Here's how the part is built. I have some questions about the finished solid (model axes, mm). A direction names the side the tool comes from. Round coordinates to 2 decimals unless told otherwise and drop trailing zeros. Order: outer loops, then holes, each group sorted by start corner. A loop starts at its lowest first (then second) coordinate and runs counter-clockwise, first axis right, second up. Notation, with made-up numbers: (-3, 5.25) -> (34, 5.25) arc R14 cw to (34, 22.25) -> close; hole circle Ø11 at (18.5, -7.5). An arc over 180 degrees is marked (long way). One line per item, written item: value.
Autodesk Inventor part; units mm, degrees
ref_plane "YZ Plane" through (0, 0, 0) normal (1, 0, 0) x (0, 1, 0)
ref_plane "XZ Plane" through (0, 0, 0) normal (0, 1, 0) x (-1, 0, 0)
ref_plane "XY Plane" through (0, 0, 0) normal (0, 0, 1) x (1, 0, 0)
sketch "Sketch1" plane through (0, 0, 0) normal (0, 0, 1) x (1, 0, 0)
  line L0 (-12.7, -12.7) -> (12.7, -12.7)
  line L1 (12.7, -12.7) -> (12.7, 12.7)
  line L2 (12.7, 12.7) -> (-12.7, 12.7)
  line L3 (-12.7, 12.7) -> (-12.7, -12.7)
  line L4 (-12.7, -12.7) -> (12.7, 12.7) construction
  line L5 (12.7, -12.7) -> (-12.7, 12.7) construction
  line L6 (-11.1125, 11.1125) -> (11.1125, 11.1125)
  line L7 (11.1125, 11.1125) -> (11.1125, -11.1125)
  line L8 (11.1125, -11.1125) -> (-11.1125, -11.1125)
  line L9 (-11.1125, -11.1125) -> (-11.1125, 11.1125)
  point P0 (0, 0)
  dimension "width" = 25.4
  dimension "height" = 25.4
  dimension "thickness" = 1.5875
extrude "Extrusion1" add sketch "Sketch1" along normal mid plane 431.8
sketch "Sketch3" plane through (-12.7, 12.7, 215.9) normal (0, 1, 0) x (1, 0, 0)
  line L0 (0, 431.8) -> (0, 0) construction
  line L1 (25.4, 0) -> (0, 0) construction
  line L2 (25.4, 431.8) -> (25.4, 0) construction
  line L3 (0, 431.8) -> (25.4, 431.8) construction
  line L4 (0, 0) -> (0, 431.8) construction
  line L5 (0, 0) -> (25.4, 17.7853)
  line L6 (25.4, 431.8) -> (25.4, 0) construction
  line L7 (0, 0) -> (25.4, 0) construction
  line L8 (0, 0) -> (25.4, 0)
  line L9 (25.4, 0) -> (25.4, 17.7853)
  line L10 (0, 431.8) -> (25.4, 395.525)
  line L11 (25.4, 431.8) -> (0, 431.8) construction
  line L12 (0, 431.8) -> (25.4, 431.8)
  line L13 (25.4, 431.8) -> (25.4, 395.525)
  point P0 (12.7, 215.9)
  dimension "d12" = 55
extrude "Extrusion3" cut sketch "Sketch3" against normal through all
sketch "Sketch4" plane through (-12.7, 12.7, 215.9) normal (0, 1, 0) x (1, 0, 0)
  line L0 (25.4, 17.7853) -> (0, 0) construction
  line L1 (0, 0) -> (0, 431.8) construction
  line L2 (0, 431.8) -> (25.4, 395.525) construction
  line L3 (25.4, 395.525) -> (25.4, 17.7853) construction
  point P0 (12.7, 215.9)
  point P1 (12.7, 19.05)
  point P2 (12.7, 31.75)
  point P3 (12.7, 44.45)
  point P4 (12.7, 57.15)
  point P5 (12.7, 400.05)
  point P6 (12.7, 387.35)
  point P7 (12.7, 374.65)
  dimension "d13" = 19.05
  dimension "d16" = 12.7
  dimension "d28" = 31.75
  dimension "d31" = 12.7
hole "Hole1" at (0, 12.7, 196.85) at (0, 12.7, 184.15) at (0, 12.7, -158.75) at (0, 12.7, -171.45) at (0, 12.7, -184.15) direction (0, -1, 0) diameter 5.1054 end through all
sketch "Sketch5" plane through (-12.7, -12.7, 215.9) normal (-1, 0, 0) x (0, 0, 1)
  line L0 (-431.8, 0) -> (-431.8, 25.4) construction
  point P0 (-215.9, 12.7)
  point P1 (-241.3, 12.7)
  point P2 (-203.2, 12.7)
  point P3 (-431.8, 12.7)
  dimension "d36" = 38.1
  dimension "d37" = 190.5
hole "Hole2" at (-12.7, 0, -25.4) at (-12.7, 0, 12.7) direction (1, 0, 0) diameter 5.1054 end through all
sketch "Sketch6" plane through (-12.7, 12.7, 215.9) normal (0, 1, 0) x (1, 0, 0)
  line L0 (25.4, 395.525) -> (25.4, 17.7853) construction
  circle A0 centre (12.7, 374.65) radius 2.5527 construction
  point P0 (12.7, 215.9)
  point P1 (12.7, 222.25)
  point P2 (12.7, 190.5)
  dimension "d45" = 31.75
  dimension "d46" = 12.7
  dimension "d47" = 152.4
hole "Hole3" at (0, 12.7, -6.35) at (0, 12.7, 25.4) direction (0, -1, 0) diameter 5.1054 end through all
properties part number "CL-002" material "Aluminum 6061"
Q1. If we mould it in two halves opening along X, with no side actions, what happens to faces 1 (the face through (0, 12.7, -3)), 2 (the face through (11.112, 0, 6)), 3 (the face through (12.7, 0, 7))? For each: pulls with the +X half, pulls with the -X half, needs draft (parallel to the pull), parting line crosses it, or undercut.
Answers:
face 1: needs draft
face 2: undercut
face 3: pulls with the +X half
Q2. I need wall thicknesses on line 1 along Y through (x, z) = (-6, 48.5); line 2 along Y through (x, z) = (11.5, -25.4). Which ranges of each line are inside material? Lowest first, please.
Answers:
line 1: -12.7 to -11.11, 11.11 to 12.7
line 2: -12.7 to -2.55, 2.55 to 12.7
Q3. I want a section at A-A on y = -7. Write out the boundary of the cut face in (x, z) (1 decimal), then the cut area to 3 significant figures.
Answers:
outline: (-12.7, -215.9) -> (-11.1, -213.6) -> (-11.1, 214.8) -> (-12.7, 215.9) -> close; (11.1, -181.9) -> (12.7, -179.6) -> (12.7, 198.1) -> (11.1, 199.2) -> close
area: 1,290 mm2
Q4. Which directions (+Z, -Z, +X, -X, +Y, -Y) give clear straight access to the entire face, cutting with the end or side of a thin tool? Please do faces 4 (the face through (-0.06, 11.35, -197.85)), 5 (the face through (0, -11.112, -2)).
Answers:
face 4: -Z, +X, +Y, -Y
face 5: +Z, -Z
Q5. I want a section at B-B on z = -130.5. Write out the boundary of the cut face in (x, y).
Answers:
outline: (-12.7, -12.7) -> (12.7, -12.7) -> (12.7, 12.7) -> (-12.7, 12.7) -> close; hole (-11.11, -11.11) -> (11.11, -11.11) -> (11.11, 11.11) -> (-11.11, 11.11) -> close
